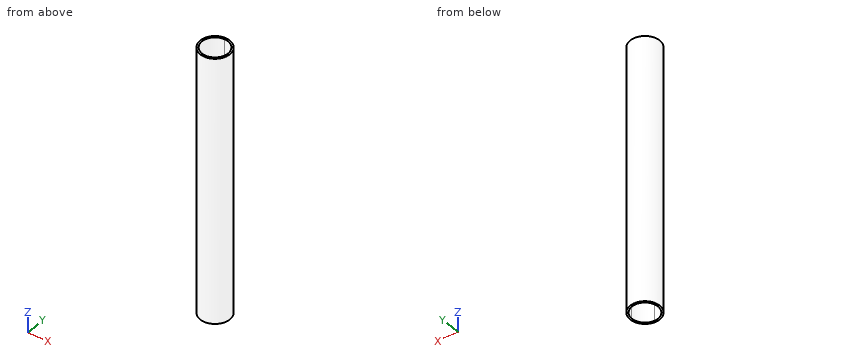
```python
from build123d import *

# Parameters (mm, degrees)
F0_R     = 8.0645
F1_DEPTH = 72.5551
F2_DEPTH = 72.5551
F3_DEPTH = 25.4
F5_DEPTH = 145.1102


with BuildPart() as f1:
    # F0 (on Top) → F1 (new body)
    with BuildSketch(Plane.XY):
        Circle(F0_R)
    extrude(amount=F1_DEPTH)

    # F0 (on Top) → F2 (join)
    with BuildSketch(Plane.XY):
        Circle(F0_R)
    extrude(amount=-F2_DEPTH)

    # F0 (on Top) → F3 (join)
    with BuildSketch(Plane.XY):
        Circle(F0_R)
    extrude(amount=F3_DEPTH)

    # F4 (on face) → F5 (cut)
    with BuildSketch(Plane(origin=(0, 0, -72.5551), x_dir=(1, 0, 0), z_dir=(0, 0, -1))):
        with BuildLine():
            Line((0, -7.0866), (0, 7.0866))
            ThreePointArc((0, 7.0866), (-7.0866, 0), (0, -7.0866))
        make_face()
        with BuildLine():
            ThreePointArc((0, -7.0866), (5.010983, -5.010983), (7.0866, 0))
            ThreePointArc((7.0866, 0), (5.010983, 5.010983), (0, 7.0866))
            Line((0, 7.0866), (0, -7.0866))
        make_face()
    extrude(amount=-F5_DEPTH, mode=Mode.SUBTRACT)


solid = f1.part
```
Could you check a few things on this model? Use its own coordinates, in mm. Coordinates: 2 decimals unless noted, no trailing zeros. Write each loop counter-clockwise with the first axis right and the second up, starting at its lowest first coordinate (ties: lowest second). Pieces come first, ordered by that corner, then holes. Notation, with made-up numbers: (36, 4) -> (62, 4) arc R31 cw to (62, 43) -> close; hole circle Ø11 at (45.5, -20). An arc over 180 degrees is marked (long way). One line per question, with ' | ' between items. Start each with the question number.
1. If we section it at A-A (x = -1.5): Please give me the cut outline in (y, z), and give its area (3 significant figures).
2. Will these pins go through, and if not, where does the flat tip stop? P1, Ø2, axis at y = -6.5, z = -4, coming from the +X side; P2, Ø5, axis at y = 4, z = 24.5, coming from the -X side; P3, Ø5, axis at y = -6, z = -42, coming from the +X side.
3. Please list where these lines run through material, in increasing order: line 1 along Y through (x, z) = (0.5, -39); line 2 along Y through (x, z) = (0.25, -55).
4. If we section it at B-B (y = -5): Please give me the cut outline in (x, z).
5. If we section it at C-C (z = -32): Please give me the cut outline in (x, y), and give its area (3 significant figures).
Return value:
1) outline: (-7.92, -72.56) -> (-6.93, -72.56) -> (-6.93, 72.56) -> (-7.92, 72.56) -> close; (6.93, -72.56) -> (7.92, -72.56) -> (7.92, 72.56) -> (6.93, 72.56) -> close | area: 290 mm²
2) P1: stops at x = 5.9 | P2: stops at x = -7.92 | P3: stops at x = 7.27
3) line 1: y = -8.05 to -7.07, 7.07 to 8.05 | line 2: y = -8.06 to -7.08, 7.08 to 8.06
4) outline: (-6.33, -72.56) -> (-5.02, -72.56) -> (-5.02, 72.56) -> (-6.33, 72.56) -> close; (5.02, -72.56) -> (6.33, -72.56) -> (6.33, 72.56) -> (5.02, 72.56) -> close
5) outline: circle Ø16.13 at (0, 0); hole circle Ø14.17 at (0, 0) | area: 46.5 mm²
